Could you check a few things on this drawing? It's one solid part, dimensions in mm from its lowest x, y, z. A direction names the side the tool comes from. Give positions to 0.01 mm unless a question says otherwise; leave off trailing zeros. Loops run counter-clockwise (first coordinate to the right, second up) from the corner with the lowest first, then second, coordinate; pieces in that order, holes last. Notation, with made-up numbers: (-2.5, 20.5) - (40.5, 20.5) arc R21 cw to (40.5, 29.5) - close; hole circle Ø4 at (64, 20.25). An arc over 180 degrees is marked (long way). Write each question's results on one line, items separated by ' | '. Start each with the question number.
(1) I need wall thicknesses on line 1 (Y direction, x = 4.75, z = 7.5); line 2 (Z direction, x = 6.75, y = 9.75); line 3 (X direction, y = 13.5, z = 13.75). Which ranges of each line are inside material? Lowest first, please.
(2) On a 3-axis mill with a long thin cutter (end or side, diameter ignored), from which of +Z, -Z, +X, -X, +Y, -Y can I reach the whole of each face in a straight line? I mean the marked faces 1, 2 and 3. Say none if no direction works.
(3) Suppose I cut it at A-A (x = 9). Please give me the cut outline in (y, z) (3 decimals), and give its area (3 significant figures).
(4) Suppose I cut it at B-B (x = 5.75). Please give me the cut outline in (y, z) (3 decimals).
(5) For pin 1 (2 mm diameter, centred on y = 15, z = 6, fed in from -X); pin 2 (6 mm diameter, centred on x = 1, y = 12, fed in from -Z); pin 3 (4 mm diameter, centred on x = 5.5, z = 4, fed in from +Y); pin 4 (5 mm diameter, centred on x = 5, z = 9.5, fed in from -Y), each with a flat end and sliding along its axis, tell me the tip position at first contact or that it passes through.
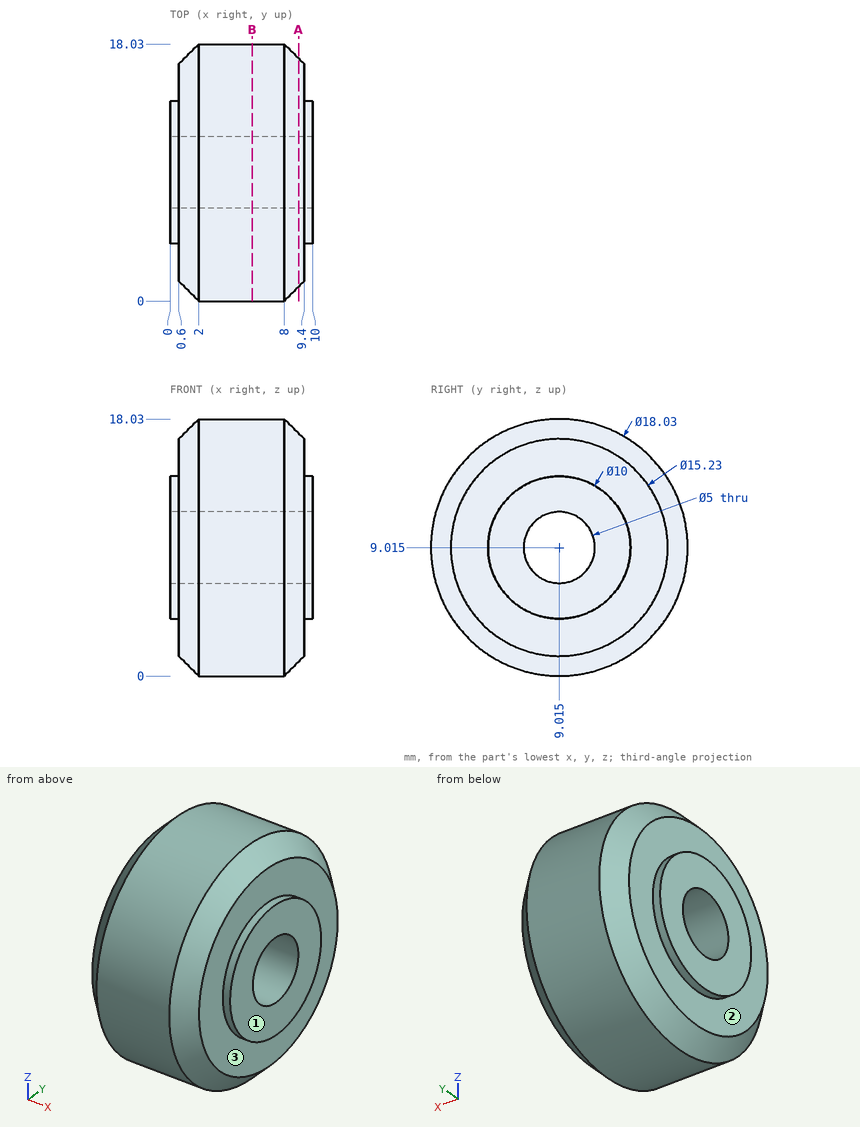
Output values:
1) line 1: 0.13 to 7.03, 11 to 17.9 | line 2: 0.03 to 6.63, 11.4 to 18 | line 3: 0.6 to 9.4
2) face 1: +Z, -Z, +X, +Y, -Y | face 2: -X | face 3: +X
3) outline: circle Ø16.03 at (9.015, 9.015); hole circle Ø5 at (9.015, 9.015) | area: 182 mm2
4) outline: circle Ø18.03 at (9.015, 9.015); hole circle Ø5 at (9.015, 9.015)
5) pin 1: x = 0.6 | pin 2: z = 0 | pin 3: y = 17.51 | pin 4: y = 0
